```python
from build123d import *

# Parameters (mm, degrees)
SKETCH_1_W          = 22.5
SKETCH_1_H          = 22.5
EXTRUDE_1_DEPTH     = 45
SKETCH_2_W          = 20.5
SKETCH_2_H          = 20.5
CUT_EXTRUDE_1_DEPTH = 40
SKETCH_3_R          = 5
CUT_EXTRUDE_2_DEPTH = 40


with BuildPart() as part:
    # 草图1 → 凸台-拉伸1 (new body)
    with BuildSketch(Plane(origin=(0, 0, 0), x_dir=(1, 0, 0), z_dir=(0, 1, 0))):
        with Locations((-11.25, -11.25)):
            Rectangle(SKETCH_1_W, SKETCH_1_H)
    extrude(amount=EXTRUDE_1_DEPTH)

    # 草图2 → 切除-拉伸1 (cut)
    with BuildSketch(Plane(origin=(0, 45, 0), x_dir=(1, 0, 0), z_dir=(0, 1, 0))):
        with Locations((-11.25, -11.25)):
            Rectangle(SKETCH_2_W, SKETCH_2_H)
    extrude(amount=-CUT_EXTRUDE_1_DEPTH, mode=Mode.SUBTRACT)

    # 草图3 → 切除-拉伸2 (cut)
    with BuildSketch(Plane.ZY.offset(22.5)):
        with Locations((11.036111031, 25)):
            Circle(SKETCH_3_R)
    extrude(amount=-CUT_EXTRUDE_2_DEPTH, mode=Mode.SUBTRACT)


solid = part.part
```
Model file for the job. Use its own axes, mm. A direction names the side the tool comes from. Coordinates: 2 decimals unless noted, no trailing zeros. Order: outer loops, then holes, each group sorted by start corner. A loop starts at its lowest first (then second) coordinate and runs counter-clockwise, first axis right, second up. Notation, with made-up numbers: (-22.5, 18) -> (35.5, 18) arc R18 cw to (35.5, 49) -> close; hole circle Ø9 at (-0.75, -30.5). An arc over 180 degrees is marked (long way). Answer as a JSON object with one key per item and string values. Group by question number.
1) Flat gauge pins, fed straight in: pin 1 (4 mm diameter, centred on x = -18, z = 5.5, fed in from +Y); pin 2 (9 mm diameter, centred on y = 25, z = 11.04, fed in from +X). Where does each tip first touch, or does it go through?
2) Cut at A-A, the plane y = 7.5. Write the cut outline in (x, z), then the cut area to 3 significant figures.
3) Cut at D-D, the plane z = 17. Write the cut outline in (x, y).
4) Cut at B-B, the plane x = -7.5. Write the cut outline in (y, z).
5) Cut at C-C, the plane y = 25. Write the cut outline in (x, z), then the cut area to 3 significant figures.
6) Which spindle directions (+Z, -Z, +X, -X, +Y, -Y) get a long thin tool onto all of the face, cutting with end or side? Do faces 1 (the face through (-11, 22, 22.5)), 2 (the face through (-11, 25, 21.5)). Say none if no direction does.
7) Pull direction X, two halves, no side cores. Call faces 3 (the face through (-11, 25, 1)), 4 (the face through (-22.5, 17, 11)), 5 (the face through (-11, 0, 11)): +X half, -X half, draft (parallel to the pull), parting line (faces both ways), or undercut.
8) Drill centre lines: L1, parallel to X at y = 11, z = 21; L2, parallel to Z at x = -12, y = 5.5; L3, parallel to Y at x = -13.5, z = 15.75. Where is each one in solid material? Low to high.
Check values:
{
 "1": {"pin 1": "stops at y = 5", "pin 2": "passes through"},
 "2": {"outline": "(-22.5, 0) -> (0, 0) -> (0, 22.5) -> (-22.5, 22.5) -> close; hole (-21.5, 1) -> (-1, 1) -> (-1, 21.5) -> (-21.5, 21.5) -> close", "area": "86.0 mm²"},
 "3": {"outline": "(-22.5, 0) -> (0, 0) -> (0, 45) -> (-1, 45) -> (-1, 5) -> (-21.5, 5) -> (-21.5, 45) -> (-22.5, 45) -> close"},
 "4": {"outline": "(0, 0) -> (45, 0) -> (45, 1) -> (5, 1) -> (5, 21.5) -> (45, 21.5) -> (45, 22.5) -> (0, 22.5) -> close"},
 "5": {"outline": "(-22.5, 0) -> (0, 0) -> (0, 6.04) -> (-1, 6.04) -> (-1, 1) -> (-21.5, 1) -> (-21.5, 6.04) -> (-22.5, 6.04) -> close; (-22.5, 16.04) -> (-21.5, 16.04) -> (-21.5, 21.5) -> (-1, 21.5) -> (-1, 16.04) -> (0, 16.04) -> (0, 22.5) -> (-22.5, 22.5) -> close", "area": "66.0 mm²"},
 "6": {"face 1": "+Z, +X, -X, +Y, -Y", "face 2": "+Y"},
 "7": {"face 3": "undercut", "face 4": "-X half", "face 5": "draft"},
 "8": {"L1": "x = -22.5 to -21.5, -1 to 0", "L2": "z = 0 to 1, 21.5 to 22.5", "L3": "y = 0 to 5"}
}
